Here's how the part is built. I have some questions about the finished solid (model axes, mm). A direction names the side the tool comes from. Round coordinates to 2 decimals unless told otherwise and drop trailing zeros. Order: outer loops, then holes, each group sorted by start corner. A loop starts at its lowest first (then second) coordinate and runs counter-clockwise, first axis right, second up.
Autodesk Inventor part; units mm, degrees
ref_plane "YZ Plane" through (0, 0, 0) normal (1, 0, 0) x (0, 1, 0)
ref_plane "XZ Plane" through (0, 0, 0) normal (0, 1, 0) x (-1, 0, 0)
ref_plane "XY Plane" through (0, 0, 0) normal (0, 0, 1) x (1, 0, 0)
sketch "Sketch1" plane through (0, 0, 0) normal (0, 1, 0) x (-1, 0, 0)
  line L0 (24.7933, -42.1134) -> (-6.7642, -42.1134)
  line L1 (-6.7642, -42.1134) -> (-6.7642, 45.097)
  line L2 (-6.7642, 45.097) -> (24.7933, 45.097)
  line L3 (24.7933, 45.097) -> (24.7933, -42.1134)
  line L4 (21.7933, -39.1134) -> (-3.7642, -39.1134)
  line L5 (-3.7642, -39.1134) -> (-3.7642, 42.097)
  line L6 (-3.7642, 42.097) -> (21.7933, 42.097)
  line L7 (21.7933, 42.097) -> (21.7933, -39.1134)
  point P0 (0, 0)
  dimension "d0" = 3
  dimension "d1" = 3
  dimension "d2" = 3
  dimension "d3" = 3
extrude "Extrusion2" add sketch "Sketch1" against normal blind 3 contours L0 L1 L2 L3 | L4 L5 L6 L7
extrude "Extrusion3" add sketch "Sketch1" along normal blind 10
properties part number "housing_bottom"
1) If we section it at C-C (x = -2): Write out the boundary of the cut face in (y, z), plus the area to 3 significant figures.
2) We'd pull the mould along X, two halves only. Please class faces 1 (the flat face through (-9, -3, 2)), 2 (the flat face through (3.764, 5, 1)), 3 (the flat face through (6.764, 3, 1)): +X half, -X half, draft (parallel to the pull), parting line (faces both ways), or undercut.
3) If we section it at B-B (z = 16.5): Write out the boundary of the cut face in (x, y).
4) I need wall thicknesses on line 1 (X direction, y = 4.25, z = 11); line 2 (Z direction, x = -9, y = 1.25); line 3 (Y direction, x = -18.5, z = 13). Which ranges of each line are inside material? Lowest first, please.
5) For faces 4 (the flat face through (-21.793, 5, 2)), 5 (the flat face through (-9, 3, 45.097)), which set-ups out of +Z, -Z, +X, -X, +Y, -Y let a thin tool reach every point of the face, with its end or its side?
6) If we section it at A-A (y = 3): Write out the boundary of the cut face in (x, z).
7) I'm going to push a flat-ended pin straight in: pin 1 (1.5 mm diameter, centred on x = -20, z = -10, fed in from +Y). Where does the tip first touch, or does it pass through?
Solutions:
1. outline: (-3, -42.11) - (10, -42.11) - (10, -39.11) - (0, -39.11) - (0, 42.1) - (10, 42.1) - (10, 45.1) - (-3, 45.1) - close
1. area: 322 mm2
2. face 1: draft
2. face 2: undercut
2. face 3: +X half
3. outline: (-24.79, -3) - (6.76, -3) - (6.76, 10) - (3.76, 10) - (3.76, 0) - (-21.79, 0) - (-21.79, 10) - (-24.79, 10) - close
4. line 1: x = -24.79 to -21.79, 3.76 to 6.76
4. line 2: z = -42.11 to -39.11, 42.1 to 45.1
4. line 3: y = -3 to 0
5. face 4: +Y
5. face 5: +Z, +X, -X, +Y, -Y
6. outline: (-24.79, -42.11) - (6.76, -42.11) - (6.76, 45.1) - (-24.79, 45.1) - close; hole (-21.79, -39.11) - (3.76, -39.11) - (3.76, 42.1) - (-21.79, 42.1) - close
7. pin 1: stops at y = 0
